Can you work these out from the model? Positions are in its coordinate system, mm. Coordinates: 2 decimals unless noted, no trailing zeros. Order: outer loops, then holes, each group sorted by start corner. A loop starts at its lowest first (then second) coordinate and runs counter-clockwise, first axis right, second up. Notation, with made-up numbers: (-26, 52.25) -> (26, 52.25) arc R19 ccw to (26, 87.25) -> close; hole circle Ø10 at (51, -28). An arc over 180 degrees is marked (long way). Return JSON: item names as keys, results as strings. Group by question number.
1) For pin 1 (1 mm diameter, centred on x = -13, y = 1, fed in from -Z), with a flat end and sliding along its axis, tell me the tip position at first contact or that it passes through.
2) If we section it at A-A, the plane y = 2.2: Please give me the cut outline in (x, z).
3) If I drill on probe 1 along X at (y, z) = (2.1, 9.5); probe 2 along X at (y, z) = (1.9, -21.5); probe 3 along X at (y, z) = (0.05, 0), over which ranges is the centre line in solid material (lowest first)? Write a range as from..to.
from build123d import *

# Parameters (mm, degrees)
SKETCH1_R           = 27
SKETCH1_R_2         = 19.7
BOSS_EXTRUDE1_DEPTH = 2.6
FILLET1_R           = 2.6
CHAMFER1_SIZE       = 1


with BuildPart() as part:
    # Sketch1 → Boss-Extrude1 (new body)
    with BuildSketch(Plane(origin=(0, 0, 0), x_dir=(1, 0, 0), z_dir=(0, 1, 0))):
        with Locations(Location((0, 0, 0), (0, 0, 270))):
            Circle(SKETCH1_R)
        with Locations(Location((0, 0, 0), (0, 0, 270))):
            Circle(SKETCH1_R_2, mode=Mode.SUBTRACT)
    extrude(amount=BOSS_EXTRUDE1_DEPTH)

    # Fillet1
    fillet1_edges = [part.edges().sort_by_distance(p)[0] for p in [
        (0, 2.6, -19.7),
    ]]
    fillet(fillet1_edges, radius=FILLET1_R - 0.0001)  # a hair under: the kernel refuses the full size

    # Chamfer1
    chamfer1_edges = [part.edges().sort_by_distance(p)[0] for p in [
        (0, 2.6, -27),
    ]]
    chamfer(chamfer1_edges, length=CHAMFER1_SIZE)

    # Cut-Sweep1: sweep along a curve in space
    with BuildLine() as cut_sweep1_path:
        ThreePointArc((0, 0, 19.7), (13.930003589, 0, 13.930003589), (19.7, 0, 0))
        ThreePointArc((19.7, 0, 0), (13.930003589, 0, -13.930003589), (0, 0, -19.7))
        ThreePointArc((0, 0, -19.7), (-13.930003589, 0, -13.930003589), (-19.7, 0, 0))
        ThreePointArc((-19.7, 0, 0), (-13.930003589, 0, 13.930003589), (0, 0, 19.7))
    # Sketch2 → Cut-Sweep1 (sweep, cut)
    with BuildSketch(Plane(origin=(0, 0, 0), x_dir=(0, 0, -1), z_dir=(1, 0, 0))):
        Polygon((24.5, 2.6), (24, 1.733974596), (23.5, 2.6), align=None)
    sweep(path=cut_sweep1_path.line, mode=Mode.SUBTRACT)


solid = part.part
Result sheet:
{
 "1": {"pin 1": "stops at z = -23.93"},
 "2": {"outline": "circle Ø52.8 at (0, 0); circle Ø47.46 at (0, 0); hole circle Ø48.54 at (0, 0); hole circle Ø41.83 at (0, 0)"},
 "3": {"probe 1": "x = -24.74..-22.27, -21.81..-18.47, 18.47..21.81, 22.27..24.74", "probe 2": "x = -15.83..-10.88, -10.45..10.45, 10.88..15.83", "probe 3": "x = -27..-19.7, 19.7..27"}
}
